```python
from build123d import *

# Parameters (mm, degrees)
SKETCH1_R           = 6
SKETCH1_R_2         = 4
BOSS_EXTRUDE1_DEPTH = 10
SKETCH2_R           = 6
BOSS_EXTRUDE2_DEPTH = 3
SKETCH3_R           = 3.95
BOSS_EXTRUDE3_DEPTH = 20
FILLET1_R           = 1
FILLET2_R           = 10
FILLET3_R           = 1
FILLET4_R           = 10


with BuildPart() as part:
    # Sketch1 → Boss-Extrude1 (new body)
    with BuildSketch(Plane(origin=(0, 0, 0), x_dir=(1, 0, 0), z_dir=(0, 1, 0))):
        with Locations(Location((0, 0, 0), (0, 0, 270))):
            Circle(SKETCH1_R)
        with Locations(Location((0, 0, 0), (0, 0, 270))):
            Circle(SKETCH1_R_2, mode=Mode.SUBTRACT)
    extrude(amount=BOSS_EXTRUDE1_DEPTH)

    # Sketch2 → Boss-Extrude2 (add)
    with BuildSketch(Plane(origin=(0, 10, 0), x_dir=(1, 0, 0), z_dir=(0, 1, 0))):
        with Locations(Location((0, 0, 0), (0, 0, 270))):
            Circle(SKETCH2_R)
    extrude(amount=BOSS_EXTRUDE2_DEPTH)

    # Sketch3 → Boss-Extrude3 (add)
    with BuildSketch(Plane(origin=(0, 13, 0), x_dir=(1, 0, 0), z_dir=(0, 1, 0))):
        with Locations(Location((0, 0, 0), (0, 0, 270))):
            Circle(SKETCH3_R)
    extrude(amount=BOSS_EXTRUDE3_DEPTH)

    # Fillet1
    fillet1_edges = [part.edges().sort_by_distance(p)[0] for p in [
        (0, 33, -3.95),
    ]]
    fillet(fillet1_edges, radius=FILLET1_R)

    # Fillet2
    # the kernel refuses this fillet: 10 mm, written as the material it adds along each edge
    with BuildSketch(Plane(origin=(0, 13, 0), x_dir=(0, 0, 1), z_dir=(-1, 0, 0))) as fillet2_piece_1:
        with BuildLine():
            CenterArc((13.95, 6.066094295), FILLET2_R, 180, 37.344744354)
            Line((6, 0), (5.841, -0.121321886))
            ThreePointArc((5.841, -0.121321886), (4.975, -0.2), (3.95, -0.2))
            Line((3.95, -0.2), (3.75, 0))
            Line((3.75, 0), (3.75, 6.066094295))
            Line((3.75, 6.066094295), (3.95, 6.066094295))
        make_face()
    revolve(axis=Axis((0, 13, 0), (0, 1, 0)))

    # Fillet3
    fillet3_edges = [part.edges().sort_by_distance(p)[0] for p in [
        (0, 0, -4),
    ]]
    fillet(fillet3_edges, radius=FILLET3_R)

    # Fillet4
    fillet4_edges = [part.edges().sort_by_distance(p)[0] for p in [
        (0, 13, -6),
    ]]
    fillet(fillet4_edges, radius=FILLET4_R)


solid = part.part
```
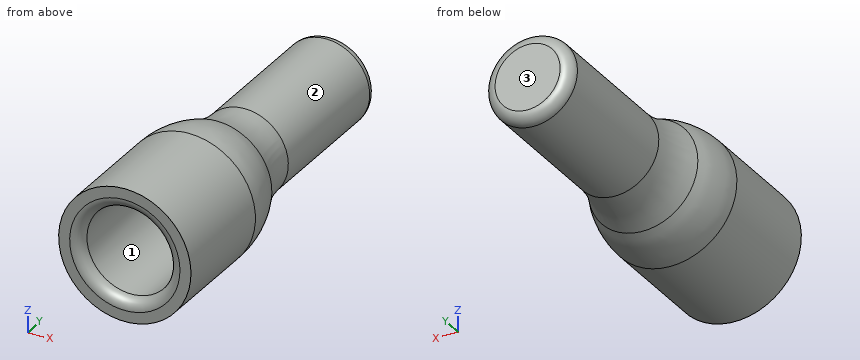
Model file for the job. Use its own axes, mm. Face numbers are marked on the shaded views. Coordinates: 2 decimals unless noted, no trailing zeros. Write each loop counter-clockwise with the first axis right and the second up, starting at its lowest first coordinate (ties: lowest second). Pieces come first, ordered by that corner, then holes. Notation, with made-up numbers: (-39, -31) - (-25, -31) arc R22 ccw to (-25, -13) - close; hole circle Ø10 at (-23, 58.25). An arc over 180 degrees is marked (long way). Use a Markdown table: item, result. Add a question column.
Item 1: Band-saw the part on B-B, the plane y = 24. Write the cut outline in (x, z), and give its area (3 significant figures).
Item 2: Band-saw the part on A-A, the plane y = 9.5. Write the cut outline in (x, z), and give its area (3 significant figures).
Item 3: Two-plate mould, pull along Z, no slides. Class the marked faces 1, 2 and 3: pulls with the +Z half, pulls with the -Z half, needs draft (parallel to the pull), parting line crosses it, or undercut.
Item 4: Band-saw the part on C-C, the plane y = 16. Write the cut outline in (x, z).
Item 5: Drill centre lines: line 1 along X through (y, z) = (6.5, 0); line 2 along Y through (x, z) = (-2, 1); line 3 along X through (y, z) = (10.5, 0). Where is each one in solid material? Low to high.
Item 6: Drop flat-ended pins along their axis: pin 1 (2 mm diameter, centred on x = -2, z = 2.5, fed in from +Y); pin 2 (5 mm diameter, centred on x = 3, y = 7, fed in from -Z); pin 3 (6 mm diameter, centred on y = 24.5, z = 1, fed in from -X); pin 4 (2.5 mm diameter, centred on x = 0.5, z = 0, fed in from -Y). Give the stop position or say it passes through.
A:
| question | item | result |
|---|---|---|
| 1 | outline | circle Ø7.9 at (0, 0) |
| 1 | area | 49.0 mm² |
| 2 | outline | circle Ø12 at (0, 0); hole circle Ø8 at (0, 0) |
| 2 | area | 62.8 mm² |
| 3 | face 1 | undercut |
| 3 | face 2 | parting line crosses it |
| 3 | face 3 | needs draft |
| 4 | outline | circle Ø8.86 at (0, 0) |
| 5 | line 1 | x = -6 to -4, 4 to 6 |
| 5 | line 2 | y = 10 to 33 |
| 5 | line 3 | x = -6 to 6 |
| 6 | pin 1 | stops at y = 33 |
| 6 | pin 2 | stops at z = -5.98 |
| 6 | pin 3 | stops at x = -3.95 |
| 6 | pin 4 | stops at y = 10 |
